from build123d import *

# Parameters (mm, degrees)
ESQUISSE1_R             = 30
BOSS_EXTRU_1_DEPTH      = 35
BOSS_EXTRU_2_START      = -2
ESQUISSE3_R             = 33
ESQUISSE3_R_2           = 30
BOSS_EXTRU_2_DEPTH      = 30
ESQUISSE4_R             = 7
ESQUISSE4_R_2           = 2
BOSS_EXTRU_3_DEPTH      = 5
ESQUISSE5_R             = 1.5
ENL_V_MAT_EXTRU_1_DEPTH = 59.335238064


with BuildPart() as part:
    # Esquisse1 → Boss.-Extru.1 (new body)
    with BuildSketch(Plane.XY):
        Circle(ESQUISSE1_R)
    extrude(amount=BOSS_EXTRU_1_DEPTH)

    # Esquisse3 → Boss.-Extru.2 (add)
    with BuildSketch(Plane(origin=(0, 0, 0), x_dir=(-1, 0, 0), z_dir=(0, 0, -1)).offset(BOSS_EXTRU_2_START)):
        Circle(ESQUISSE3_R)
        Circle(ESQUISSE3_R_2, mode=Mode.SUBTRACT)
    extrude(amount=-BOSS_EXTRU_2_DEPTH)

    # Esquisse4 → Boss.-Extru.3 (add)
    with BuildSketch(Plane(origin=(0, 0, 0), x_dir=(-1, 0, 0), z_dir=(0, 0, -1))):
        Circle(ESQUISSE4_R)
        Circle(ESQUISSE4_R_2, mode=Mode.SUBTRACT)
    extrude(amount=BOSS_EXTRU_3_DEPTH)

    # Esquisse5 → Enlèv. mat.-Extru.1 (cut, through all)
    with BuildSketch(Plane(origin=(0, 0, 0), x_dir=(1, 0, 0), z_dir=(0, 1, 0))):
        with Locations(Location((0, 2.5, 0), (0, 0, 90))):
            Circle(ESQUISSE5_R)
    extrude(amount=ENL_V_MAT_EXTRU_1_DEPTH, mode=Mode.SUBTRACT)


solid = part.part
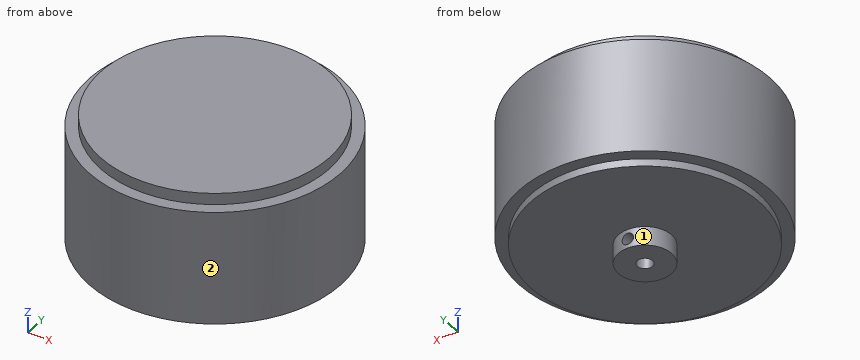
Design review of the part built by this model. Coordinates are the model's own, in mm. Face numbers are marked on the shaded views. A direction names the side the tool comes from. Give positions to 0.01 mm unless a question says otherwise; leave off trailing zeros. Order: outer loops, then holes, each group sorted by start corner. A loop starts at its lowest first (then second) coordinate and runs counter-clockwise, first axis right, second up. Notation, with made-up numbers: (66, 59) - (75, 59) arc R31 ccw to (75, 98) - close; hole circle Ø4 at (81.25, 64). An arc over 180 degrees is marked (long way). Write item = value, one per line. Start each with the question number.
Q1. To check wall thickness, follow L1, parallel to Y at x = -0.5, z = 24; L2, parallel to Y at x = 0, z = -2.6; L3, parallel to Z at x = -2.5, y = -19. State the ranges of each line that lie inside material, in increasing order. Write a range as from..to.
Q2. We need section B-B on y = 0. State the section outline as (x, z) points, plus the area to 3 significant figures.
Q3. We need section A-A on x = 0. State the section outline as (y, z) points, plus the area to 4 significant figures.
Q4. We need section C-C on x = -23. State the section outline as (y, z) points, plus the area to 3 significant figures.
Q5. We need section D-D on z = 11.5. State the section outline as (x, y) points, plus the area to 3 significant figures.
Q6. Tool access review of the marked faces 1 and 2: name each direction out of +Z, -Z, +X, -X, +Y, -Y from which nothing blocks a thin tool from reaching the whole face with its end or side.
Q7. Clearance check with flat-ended pins moving along their axes: pin 1 Ø4 at (x, y) = (-17, 3) entering from -Z; pin 2 Ø3 at (x, z) = (26, 14) entering from +Y; pin 3 Ø4 at (y, z) = (-14, 7.5) entering from -X. State where each tip first meets the part, or that it passes through.
Working result:
q1.L1 = -33..33
q1.L2 = -7..-2
q1.L3 = 0..35
q2.outline = (-33, 2) - (-30, 2) - (-30, 0) - (-7, 0) - (-7, -5) - (-2, -5) - (-2, 0) - (2, 0) - (2, -5) - (7, -5) - (7, 0) - (30, 0) - (30, 2) - (33, 2) - (33, 32) - (30, 32) - (30, 35) - (-30, 35) - (-30, 32) - (-33, 32) - close
q2.area = 2,330 mm²
q3.outline = (-33, 2) - (-30, 2) - (-30, 0) - (-7, 0) - (-7, -5) - (-2, -5) - (-2, 0) - (2, 0) - (2, -1) - (7, -1) - (7, 0) - (30, 0) - (30, 2) - (33, 2) - (33, 32) - (30, 32) - (30, 35) - (-30, 35) - (-30, 32) - (-33, 32) - close; (2, -5) - (7, -5) - (7, -4) - (2, -4) - close
q3.area = 2,315 mm²
q4.outline = (-23.66, 2) - (-19.26, 2) - (-19.26, 0) - (19.26, 0) - (19.26, 2) - (23.66, 2) - (23.66, 32) - (19.26, 32) - (19.26, 35) - (-19.26, 35) - (-19.26, 32) - (-23.66, 32) - close
q4.area = 1,610 mm²
q5.outline = circle Ø66 at (0, 0)
q5.area = 3,420 mm²
q6.face_1 = -Z
q6.face_2 = +Z, -Z
q7.pin_1 = 0
q7.pin_2 = 22.11
q7.pin_3 = -30.74
